Design review of the part shown in the three views and the two pictorial views. Dimensions are in mm from the part's minimum x, y and z. Coordinates: 2 decimals unless noted, no trailing zeros. Write each loop counter-clockwise with the first axis right and the second up, starting at its lowest first coordinate (ties: lowest second). Pieces come first, ordered by that corner, then holes. Notation, with made-up numbers: (2, 70) - (45, 70) arc R17 ccw to (45, 96) - close; hole circle Ø5 at (82.25, 69.5). An arc over 180 degrees is marked (long way). Return JSON: item names as keys, results as strings. Group by question number.
(1) Draft analysis for pull direction Y (two halves, no side actions). For the marked faces 1, 2 and 3, state which applies: released by +Y, released by -Y, zero draft, split by the parting line, or undercut.
(2) For pin 1 Ø1 at (y, z) = (3, 11.5) entering from -X; pin 2 Ø1 at (x, y) = (2.5, 2.5) entering from -Z; pin 3 Ø3 at (y, z) = (4, 7) entering from +X, all flat-tipped, find the tip position at first contact; note any pin that passes through.
(3) We need section B-B on z = 7.75. State the section outline as (x, y) points.
(4) To check wall thickness, follow L1, parallel to Y at x = 2.65, z = 8; L2, parallel to Z at x = 3.7, y = 4.2; L3, parallel to Y at x = 1.4, z = 12.75 (1 decimal). State the ranges of each line that lie inside material, in increasing order. Write a range as from..to.
(5) We need section A-A on y = 2.75. State the section outline as (x, z) points.
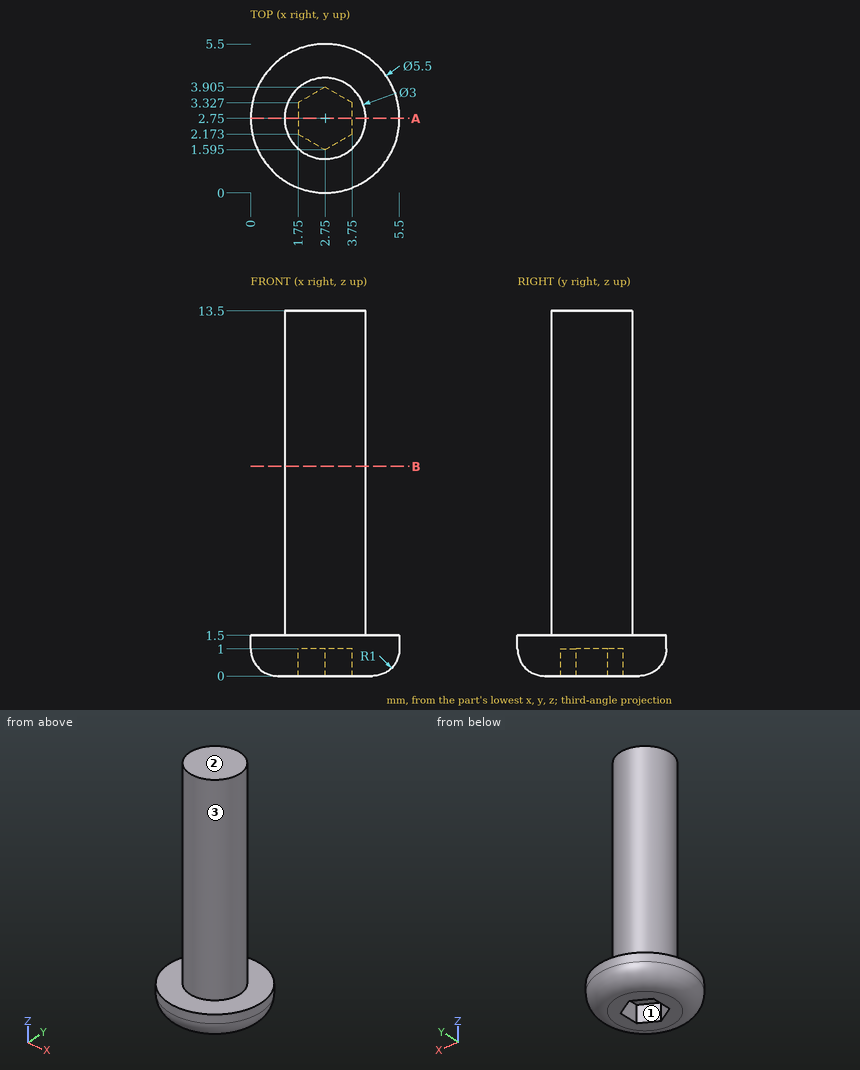
Ans:
{
 "1": {"face 1": "undercut", "face 2": "zero draft", "face 3": "split by the parting line"},
 "2": {"pin 1": "x = 1.25", "pin 2": "z = 1", "pin 3": "x = 4.25"},
 "3": {"outline": "circle Ø3 at (2.75, 2.75)"},
 "4": {"L1": "1.25..4.25", "L2": "0..1.5", "L3": "2.1..3.4"},
 "5": {"outline": "(0, 1) arc R1 ccw to (1, 0) - (1.75, 0) - (1.75, 1) - (3.75, 1) - (3.75, 0) - (4.5, 0) arc R1 ccw to (5.5, 1) - (5.5, 1.5) - (4.25, 1.5) - (4.25, 13.5) - (1.25, 13.5) - (1.25, 1.5) - (0, 1.5) - close"}
}
